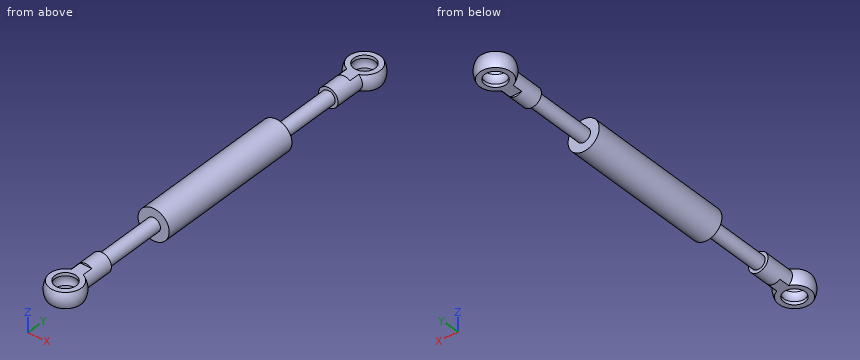
```python
from build123d import *
from build123d.topology import SkipClean

# Parameters (mm, degrees)
SKETCH_1_W               = 1.75
SKETCH_1_H               = 39
SKETCH_1_W_2             = 2.25
SKETCH_1_H_2             = 16.5
CUT_EXTRUDE_1_DEPTH      = 53.38797572
CUT_EXTRUDE_1_DEPTH_BACK = 53.38797572
SKETCH_3_W               = 3
SKETCH_3_H               = 15
CUT_EXTRUDE_2_DEPTH      = 53.538081427
CUT_EXTRUDE_2_DEPTH_BACK = 53.538081427
SKETCH_4_R               = 2.75


with BuildPart() as part:
    # Sketch 1 → Revolve 1 (revolve)
    with SkipClean():  # the faces are left unmerged after this step: merging them gives an invalid solid
        with BuildSketch(Plane.XY):
            with Locations((0.875, 0)):
                Rectangle(SKETCH_1_W, SKETCH_1_H)
            with Locations((2.875, 0)):
                Rectangle(SKETCH_1_W_2, SKETCH_1_H)
            with Locations((0.875, 27.75)):
                Rectangle(SKETCH_1_W, SKETCH_1_H_2)
            with Locations((0.875, -27.75)):
                Rectangle(SKETCH_1_W, SKETCH_1_H_2)
            Polygon((1.75, -36), (0, -36), (0, -43), (2.5, -43), (2.5, -36), align=None)
            with BuildLine():
                Line((2.5, -43), (0, -43))
                ThreePointArc((0, -43), (1.30624304, -43.19375696), (2.5, -43.758342613))
                Line((2.5, -43.758342613), (2.5, -43))
            make_face()
            with BuildLine():
                ThreePointArc((2.5, -43.758342613), (1.30624304, -43.19375696), (0, -43))
                Line((0, -43), (0, -52))
                ThreePointArc((0, -52), (3.181980515, -50.681980515), (4.5, -47.5))
                ThreePointArc((4.5, -47.5), (3.968626967, -45.378679656), (2.5, -43.758342613))
            make_face()
            with BuildLine():
                Line((0, -52), (0, -43))
                ThreePointArc((0, -43), (-1.30624304, -43.19375696), (-2.5, -43.758342613))
                ThreePointArc((-2.5, -43.758342613), (-4.30624304, -48.80624304), (0, -52))
            make_face()
            Polygon((2.5, 36), (2.5, 43), (0, 43), (0, 36), (1.75, 36), align=None)
            with BuildLine():
                Line((0, 43), (2.5, 43))
                Line((2.5, 43), (2.5, 43.758342613))
                ThreePointArc((2.5, 43.758342613), (1.30624304, 43.19375696), (0, 43))
            make_face()
            with BuildLine():
                ThreePointArc((0, 43), (1.30624304, 43.19375696), (2.5, 43.758342613))
                ThreePointArc((2.5, 43.758342613), (3.968626967, 45.378679656), (4.5, 47.5))
                ThreePointArc((4.5, 47.5), (3.181980515, 50.681980515), (0, 52))
                Line((0, 52), (0, 43))
            make_face()
            with BuildLine():
                ThreePointArc((-2.5, 43.758342613), (-1.30624304, 43.19375696), (0, 43))
                Line((0, 43), (0, 52))
                ThreePointArc((0, 52), (-4.30624304, 48.80624304), (-2.5, 43.758342613))
            make_face()
        revolve(axis=Axis((0, -1000, 0), (0, 1, 0)))
    add(part.part.scale(1), mode=Mode.REPLACE)  # the faces are merged on a copy

    # Sketch 2 → Cut-Revolve 1 (revolve, cut)
    with SkipClean():  # the faces are left unmerged after this step: merging them gives an invalid solid
        with BuildSketch(Plane.XY):
            with BuildLine():
                ThreePointArc((0, -44.5), (-3, -47.5), (0, -50.5))
                Line((0, -50.5), (0, -44.5))
            make_face()
            with BuildLine():
                Line((0, -44.5), (0, -50.5))
                ThreePointArc((0, -50.5), (2.121320344, -49.621320344), (3, -47.5))
                ThreePointArc((3, -47.5), (2.121320344, -45.378679656), (0, -44.5))
            make_face()
            with BuildLine():
                ThreePointArc((0, 50.5), (-3, 47.5), (0, 44.5))
                Line((0, 44.5), (0, 50.5))
            make_face()
            with BuildLine():
                Line((0, 50.5), (0, 44.5))
                ThreePointArc((0, 44.5), (2.121320344, 45.378679656), (3, 47.5))
                ThreePointArc((3, 47.5), (2.121320344, 49.621320344), (0, 50.5))
            make_face()
        revolve(axis=Axis((0, -1000, 0), (0, 1, 0)), mode=Mode.SUBTRACT)
    add(part.part.scale(1), mode=Mode.REPLACE)  # the faces are merged on a copy

    # Sketch 3 → Cut-Extrude 1 (cut, two sides: drawn at the far end of the back side and taken through both)
    with BuildSketch(Plane(origin=(0, 0, 0), x_dir=(0, 0, -1), z_dir=(1, 0, 0)).offset(-CUT_EXTRUDE_1_DEPTH_BACK)):
        with Locations((-3.5, 48.5)):
            Rectangle(SKETCH_3_W, SKETCH_3_H)
        with Locations((3.5, 48.5)):
            Rectangle(SKETCH_3_W, SKETCH_3_H)
        with Locations((3.5, -48.5)):
            Rectangle(SKETCH_3_W, SKETCH_3_H)
        with Locations((-3.5, -48.5)):
            Rectangle(SKETCH_3_W, SKETCH_3_H)
    extrude(amount=CUT_EXTRUDE_1_DEPTH + CUT_EXTRUDE_1_DEPTH_BACK, mode=Mode.SUBTRACT)

    # Sketch 4 → Cut-Extrude 2 (cut, two sides: drawn at the far end of the back side and taken through both)
    with BuildSketch(Plane.XY.offset(2).offset(-CUT_EXTRUDE_2_DEPTH_BACK)):
        with Locations((0, 47.5)):
            Circle(SKETCH_4_R)
        with Locations((0, -47.5)):
            Circle(SKETCH_4_R)
    extrude(amount=CUT_EXTRUDE_2_DEPTH + CUT_EXTRUDE_2_DEPTH_BACK, mode=Mode.SUBTRACT)


solid = part.part
```
For this review, take the finished solid that the model builds, in its own axes (mm). Round coordinates to 2 decimals unless told otherwise and drop trailing zeros. Write each loop counter-clockwise with the first axis right and the second up, starting at its lowest first coordinate (ties: lowest second). Pieces come first, ordered by that corner, then holes. Notation, with made-up numbers: (79, 23) - (98, 23) arc R11 cw to (98, 39) - close; hole circle Ø4 at (85, 35.25). An arc over 180 degrees is marked (long way). Answer as CSV lines item,"result". Start each with the question number.
(1) For line 1 (Y direction, x = 0, z = 1.7); line 2 (Y direction, x = 2.5, z = 1); line 3 (Y direction, x = 0, z = 1.85), list the stretches that pass through material, from the lowest coordinate up.
(2) Add section D-D, the plane y = -15. State the section outline as (x, z) points.
(3) For pin 1 (4 mm diameter, centred on x = 2, y = -44, fed in from +Z); pin 2 (1.5 mm diameter, centred on x = -1, z = 0.5, fed in from -Y); pin 3 (1 mm diameter, centred on y = -27.5, z = -1, fed in from -X), all flat-tipped, find the tip position at first contact; note any pin that passes through.
(4) Add section B-B, the plane z = 0. State the section outline as (x, y) points.
(5) Add section A-A, the plane y = -47.5. State the section outline as (x, z) points, plus the area to 3 significant figures.
(6) Add section C-C, the plane x = 0. State how many separate pieces and enclosed holes the cut face has, plus the area to 3 significant figures.
From the geometry:
1,line 1,"y = -51.67 to -50.25, -44.75 to 44.75, 50.25 to 51.67"
1,line 2,"y = -51.11 to -48.82, -46.18 to -43.89, -19.5 to 19.5, 43.89 to 46.18, 48.82 to 51.11"
1,line 3,"y = -51.6 to -50.25, -44.75 to -36, -19.5 to 19.5, 36 to 44.75, 50.25 to 51.6"
2,outline,"circle Ø8 at (0, 0)"
3,pin 1,"stops at z = 2"
3,pin 2,"stops at y = -51.98"
3,pin 3,"stops at x = -1.68"
4,outline,"(-4, -19.5) - (-1.75, -19.5) - (-1.75, -36) - (-2.5, -36) - (-2.5, -43.76) arc R4.5 ccw (long way) to (2.5, -43.76) - (2.5, -36) - (1.75, -36) - (1.75, -19.5) - (4, -19.5) - (4, 19.5) - (1.75, 19.5) - (1.75, 36) - (2.5, 36) - (2.5, 43.76) arc R4.5 ccw (long way) to (-2.5, 43.76) - (-2.5, 36) - (-1.75, 36) - (-1.75, 19.5) - (-4, 19.5) - close; hole circle Ø6 at (0, -47.5); hole circle Ø6 at (0, 47.5)"
5,outline,"(-4.03, -2) - (-2.75, -2) - (-2.75, -1.2) arc R3 cw to (-2.75, 1.2) - (-2.75, 2) - (-4.03, 2) arc R4.5 ccw to start; (2.75, -2) - (4.03, -2) arc R4.5 ccw to (4.03, 2) - (2.75, 2) - (2.75, 1.2) arc R3 cw to (2.75, -1.2) - close"
5,area,"12.0 mm²"
6,separate pieces,"3"
6,enclosed holes,"0"
6,area,"519 mm²"
